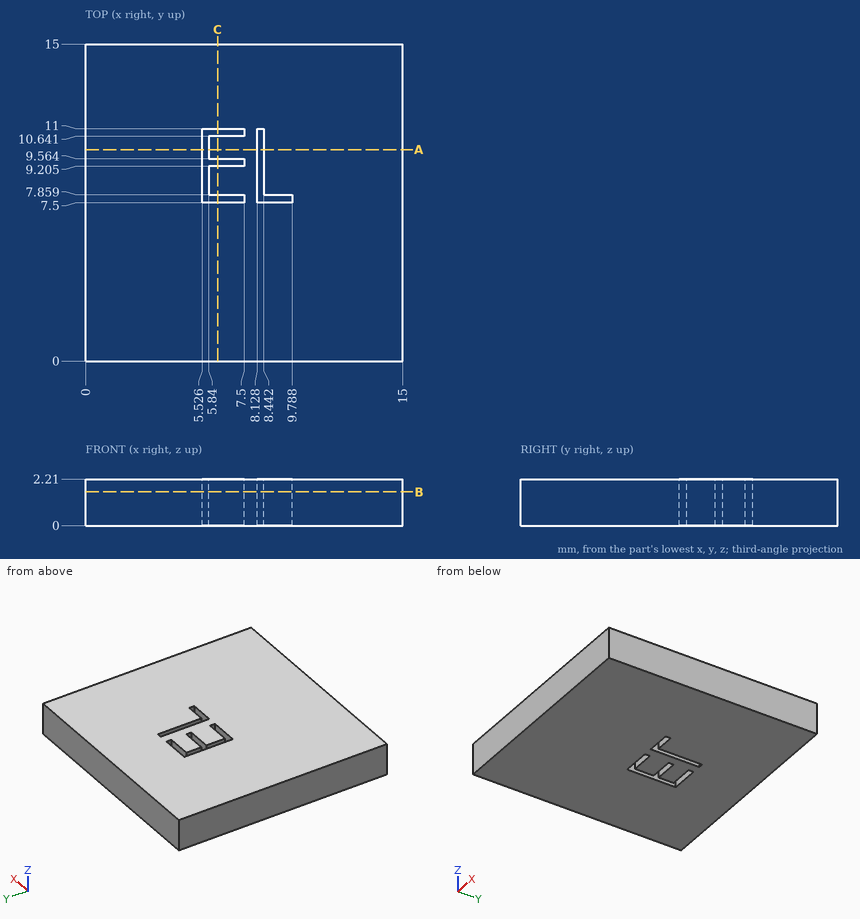
Input: dimensioned drawing with shaded views. Units: mm. Origin: part minimum x, y, z. Coordinates: 2 decimals unless noted, no trailing zeros. Order: outer loops, then holes, each group sorted by start corner. A loop starts at its lowest first (then second) coordinate and runs counter-clockwise, first axis right, second up.
(1) Section query A-A (y = 10). Return the cut outline in (x, z) (1 decimal).
(2) Section query C-C (x = 6.25). Return the cut outline in (y, z) (1 decimal).
(3) Section query B-B (z = 1.6). State how many separate pieces and enclosed holes the cut face has.
(4) Material intervals for probe 1 along Y at (x, z) = (7, 2.1) (1 decimal); probe 2 along X at (y, z) = (9, 1.25) (1 decimal); probe 3 along Y at (x, z) = (9.75, 0.7), sorted ascending.
Solution:
1. outline: (0, 0) - (5.5, 0) - (5.5, 2.2) - (0, 2.2) - close; (5.8, 0) - (8.1, 0) - (8.1, 2.2) - (5.8, 2.2) - close; (8.4, 0) - (15, 0) - (15, 2.2) - (8.4, 2.2) - close
2. outline: (0, 0) - (7.5, 0) - (7.5, 2.2) - (0, 2.2) - close; (7.9, 0) - (9.2, 0) - (9.2, 2.2) - (7.9, 2.2) - close; (9.6, 0) - (10.6, 0) - (10.6, 2.2) - (9.6, 2.2) - close; (11, 0) - (15, 0) - (15, 2.2) - (11, 2.2) - close
3. separate pieces: 1
3. enclosed holes: 2
4. probe 1: y = 0 to 7.5, 7.9 to 9.2, 9.6 to 10.6, 11 to 15
4. probe 2: x = 0 to 5.5, 5.8 to 8.1, 8.4 to 15
4. probe 3: y = 0 to 7.5, 7.86 to 15
